from build123d import *

# Parameters (mm, degrees)
SKETCH1_R           = 1.65
SKETCH1_R_2         = 2.7
BOSS_EXTRUDE1_DEPTH = 6.35


with BuildPart() as part:
    # Sketch1 → Boss-Extrude1 (new body)
    with BuildSketch(Plane.XY.offset(222.25)):
        with BuildLine():
            Line((-25.4, 57.15), (-25.4, 50.8))
            Line((-25.4, 50.8), (-50.8, 50.8))
            Line((-50.8, 50.8), (-50.8, 57.15))
            Line((-50.8, 57.15), (-325.12, 57.15))
            Line((-325.12, 57.15), (-325.12, 50.8))
            Line((-325.12, 50.8), (-350.52, 50.8))
            Line((-350.52, 50.8), (-350.52, 57.15))
            Line((-350.52, 57.15), (-382.27, 57.15))
            Line((-382.27, 57.15), (-382.27, 34.925))
            Line((-382.27, 34.925), (-375.92, 34.925))
            Line((-375.92, 34.925), (-375.92, 22.225))
            Line((-375.92, 22.225), (-382.27, 22.225))
            Line((-382.27, 22.225), (-382.27, 0))
            Line((-382.27, 0), (-320.61896879, 0))
            ThreePointArc((-320.61896879, 0), (-318.881506462, 0.306361486), (-317.353607733, 1.188494229))
            Line((-317.353607733, 1.188494229), (-299.608074729, 16.078764428))
            ThreePointArc((-299.608074729, 16.078764428), (-295.788327906, 18.284096284), (-291.444672086, 19.05))
            Line((-291.444672086, 19.05), (-84.475327914, 19.05))
            ThreePointArc((-84.475327914, 19.05), (-80.131672094, 18.284096284), (-76.311925271, 16.078764428))
            Line((-76.311925271, 16.078764428), (-58.566392267, 1.188494229))
            ThreePointArc((-58.566392267, 1.188494229), (-57.038493538, 0.306361486), (-55.30103121, 0))
            Line((-55.30103121, 0), (6.35, 0))
            Line((6.35, 0), (6.35, 22.225))
            Line((6.35, 22.225), (0, 22.225))
            Line((0, 22.225), (0, 34.925))
            Line((0, 34.925), (6.35, 34.925))
            Line((6.35, 34.925), (6.35, 57.15))
            Line((6.35, 57.15), (-25.4, 57.15))
        make_face()
        with Locations((-379.095, 11.1125)):
            Circle(SKETCH1_R, mode=Mode.SUBTRACT)
        with Locations((3.175, 11.1125)):
            Circle(SKETCH1_R, mode=Mode.SUBTRACT)
        with Locations((-379.095, 46.0375)):
            Circle(SKETCH1_R, mode=Mode.SUBTRACT)
        with Locations((3.175, 46.0375)):
            Circle(SKETCH1_R, mode=Mode.SUBTRACT)
        with Locations((-175.260005593, 41.91)):
            Circle(SKETCH1_R, mode=Mode.SUBTRACT)
        with Locations((-200.66, 41.91)):
            Circle(SKETCH1_R, mode=Mode.SUBTRACT)
        with Locations((-175.260005593, 29.21)):
            Circle(SKETCH1_R, mode=Mode.SUBTRACT)
        with Locations((-200.66, 29.21)):
            Circle(SKETCH1_R, mode=Mode.SUBTRACT)
        with Locations((-14.2875, 53.975)):
            Circle(SKETCH1_R, mode=Mode.SUBTRACT)
        with Locations((-361.6325, 53.975)):
            Circle(SKETCH1_R, mode=Mode.SUBTRACT)
        with Locations((-61.9125, 53.975)):
            Circle(SKETCH1_R, mode=Mode.SUBTRACT)
        with Locations((-314.0075, 53.975)):
            Circle(SKETCH1_R, mode=Mode.SUBTRACT)
        with Locations((-115.41, 38.26)):
            Circle(SKETCH1_R_2, mode=Mode.SUBTRACT)
        with Locations((-260.51, 38.26)):
            Circle(SKETCH1_R_2, mode=Mode.SUBTRACT)
    extrude(amount=-BOSS_EXTRUDE1_DEPTH)


solid = part.part
Design review of the part built by this model. Coordinates are the model's own, in mm. A direction names the side the tool comes from. Coordinates: 2 decimals unless noted, no trailing zeros. Loops run counter-clockwise (first coordinate to the right, second up) from the corner with the lowest first, then second, coordinate; pieces in that order, holes last. Notation, with made-up numbers: (6, 15.5) - (40, 15.5) arc R19 cw to (40, 49.5) - close; hole circle Ø9 at (18, 63). An arc over 180 degrees is marked (long way). Use CSV: the item, a comma, the result in double quotes. Start each with the question number.
1. Clearance check with a flat-ended pin moving along its axis: pin 1 (1.9 mm diameter, centred on x = -37, z = 218.5, fed in from +Y). State where the tip first meets the part, or that it passes through.
2. Mouldability with a two-part tool opening along Y and no side actions: class faces 4 (the flat face through (3, 22.225, 219)), 5 (the flat face through (3, 34.925, 219)), 6 (the flat face through (-350.52, 54, 219)), 7 (the flat face through (-67.563, 8.738, 219.119)) as released by +Y, released by -Y, zero draft, split by the parting line, or undercut.
3. Add section C-C on x = -91.5. Give the boundary of the cut face in (y, z).
4. To check wall thickness, follow probe 1 along Y at (x, z) = (-200.66, 217.5); probe 2 along X at (y, z) = (47, 221.25); probe 3 along X at (y, z) = (42, 219.25). State the ranges of each line that lie inside material, in increasing order.
5. Add section B-B on z = 218. Count the separate pieces of the cut face and the enclosed holes in it, plus the area to 3 significant figures.
6. Add section A-A on x = -39. Give the boundary of the cut face in (y, z).
7. For faces 1 (the flat face through (-308.605, 8.529, 219.119)), 2 (the flat face through (-366, 57.15, 219)), 3 (the flat face through (-325.12, 54, 219)), list the 3-axis set-ups (+Z, -Z, +X, -X, +Y, -Y) from which the entire face can be reached by the end or side of a thin tool; tool diameter is ignored.
Resolved:
1,pin 1,"y = 50.8"
2,face 4,"undercut"
2,face 5,"undercut"
2,face 6,"zero draft"
2,face 7,"released by -Y"
3,outline,"(19.05, 215.9) - (57.15, 215.9) - (57.15, 222.25) - (19.05, 222.25) - close"
4,probe 1,"19.05 to 27.56, 30.86 to 40.26, 43.56 to 57.15"
4,probe 2,"-382.27 to -380.44, -377.75 to 1.83, 4.52 to 6.35"
4,probe 3,"-382.27 to -202.31, -199.01 to -176.91, -173.61 to 6.35"
5,separate pieces,"1"
5,enclosed holes,"14"
5,area,"17,000 mm2"
6,outline,"(0, 215.9) - (50.8, 215.9) - (50.8, 222.25) - (0, 222.25) - close"
7,face 1,"+Z, -Z, -Y"
7,face 2,"+Z, -Z, +X, -X, +Y"
7,face 3,"+Z, -Z, +Y"
